```python
from build123d import *

# Parameters (mm, degrees)
F0_W     = 45.7
F0_H     = 4
F1_DEPTH = 1
F0_W_2   = 13.3
F0_H_2   = 2
F0_H_3   = 8.5
F0_W_3   = 2
F2_DEPTH = 2.5
F3_DEPTH = 5
F4_DEPTH = 8


with BuildPart() as f1:
    # F0 (on Top) → F1 (new body)
    with BuildSketch(Plane.XY):
        Polygon((59, 16.5), (59, 24.5), (45.7, 24.5), (45.7, 20.5), (45.7, 16.5), align=None)
        with Locations((22.85, 22.5)):
            Rectangle(F0_W, F0_H)
    extrude(amount=F1_DEPTH)



with BuildPart() as f1b:
    # F0 (on Top) → F1, piece 2 (new body)
    with BuildSketch(Plane.XY):
        Polygon((59, 0), (59, 8), (45.7, 8), (45.7, 4), (45.7, 0), align=None)
        with Locations((22.85, 2)):
            Rectangle(F0_W, F0_H)
    extrude(amount=F1_DEPTH)


with BuildPart() as f1_1:
    add(f1.part)

    add(f1b.part)  # F2 merges F1b
    # F0 (on Top) → F2 (join)
    with BuildSketch(Plane.XY):
        with Locations((52.35, 25.5)):
            Rectangle(F0_W_2, F0_H_2)
        with Locations((52.35, 12.25)):
            Rectangle(F0_W_2, F0_H_3)
        with Locations((52.35, -1)):
            Rectangle(F0_W_2, F0_H_2)
        with Locations((60, 12.25)):
            Rectangle(F0_W_3, F0_H_3)
        Polygon((61, -2), (61, 8), (59, 8), (59, 0), (59, -2), align=None)
        Polygon((61, 26.5), (59, 26.5), (59, 24.5), (59, 16.5), (61, 16.5), align=None)
    extrude(amount=F2_DEPTH)

    # F0 (on Top) → F3 (join)
    with BuildSketch(Plane.XY):
        Polygon((45.7, 8), (45.7, 16.5), (45.7, 20.5), (0, 20.5), (0, 4), (45.7, 4), align=None)
    extrude(amount=F3_DEPTH)

    # F0 (on Top) → F4 (join)
    with BuildSketch(Plane.XY):
        Polygon((45.7, 24.5), (45.7, 26.5), (-2, 26.5), (-2, -2), (45.7, -2), (45.7, 0), (0, 0), (0, 4), (0, 20.5), (0, 24.5), align=None)
    extrude(amount=F4_DEPTH)


solid = f1_1.part
```
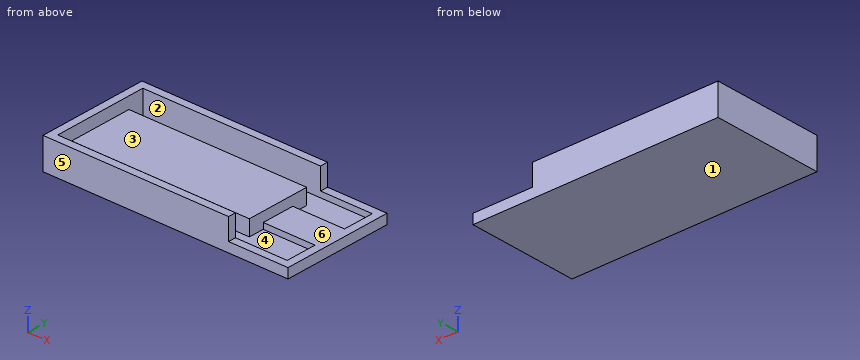
Check sheet for the modelled part. Datum: model origin and axes. Units: mm. Face numbers are marked on the shaded views. A direction names the side the tool comes from. Round coordinates to 2 decimals unless told otherwise and drop trailing zeros. Order: outer loops, then holes, each group sorted by start corner. A loop starts at its lowest first (then second) coordinate and runs counter-clockwise, first axis right, second up. Notation, with made-up numbers: M 27.25,55.5 L 43.25,55.5 A12 cw 43.25,63.5 Z; hole C -1,16.25 d6. An arc over 180 degrees is marked long. Answer in a Markdown table with one row per item.
(1) Section check A-A on z = 6.25. Record the boundary of the cut face in (x, y), plus the area to 3 significant figures.
Findings:
| item | result |
|---|---|
| outline | M -2,-2 L 45.7,-2 L 45.7,0 L 0,0 L 0,24.5 L 45.7,24.5 L 45.7,26.5 L -2,26.5 Z |
| area | 240 mm^2 |
(2) Section check D-D on x = 52.5. Record the boundary of the cut face in (y, z).
Findings:
| item | result |
|---|---|
| outline | M -2,0 L 26.5,0 L 26.5,2.5 L 24.5,2.5 L 24.5,1 L 16.5,1 L 16.5,2.5 L 8,2.5 L 8,1 L 0,1 L 0,2.5 L -2,2.5 Z |
(3) Draft check along Y on the marked faces 4, 5 and 6. Enter one of: +Y half, -Y half, draft (parallel to the pull), parting line (faces both ways), or undercut.
Findings:
| item | result |
|---|---|
| face 4 | undercut |
| face 5 | -Y half |
| face 6 | draft |
(4) Section check C-C on x = 21. Record the boundary of the cut face in (y, z).
Findings:
| item | result |
|---|---|
| outline | M -2,0 L 26.5,0 L 26.5,8 L 24.5,8 L 24.5,1 L 20.5,1 L 20.5,5 L 4,5 L 4,1 L 0,1 L 0,8 L -2,8 Z |
(5) Set-up check for the marked faces 1, 2 and 3: record each of +Z, -Z, +X, -X, +Y, -Y from which the full face is reachable in a straight line by a thin tool's end or side.
Findings:
| item | result |
|---|---|
| face 1 | -Z, +X, -X, +Y, -Y |
| face 2 | +Z |
| face 3 | +Z, +X |
(6) Section check B-B on y = 13. Record the boundary of the cut face in (x, z).
Findings:
| item | result |
|---|---|
| outline | M -2,0 L 61,0 L 61,2.5 L 45.7,2.5 L 45.7,5 L 0,5 L 0,8 L -2,8 Z |
(7) Material ranges on line 1 along Y through (x, z) = (28, 2); line 2 along Y through (x, z) = (1.5, 6); line 3 along Z through (x, y) = (54.5, 25), recorded low to high. Write a range as from..to.
Findings:
| item | result |
|---|---|
| line 1 | y = -2..0, 4..20.5, 24.5..26.5 |
| line 2 | y = -2..0, 24.5..26.5 |
| line 3 | z = 0..2.5 |
(8) Gauge pin test, flat ends, axial feed: pin 1 (1.6 mm diameter, centred on y = -0.5, z = 6, fed in from +X); pin 2 (6.5 mm diameter, centred on x = 19, y = 19, fed in from +Z); pin 3 (4 mm diameter, centred on x = 48, z = 5.5, fed in from -Y); pin 4 (7.5 mm diameter, centred on x = 56.5, y = 6, fed in from +Z). Record the tip position at first contact, or that the pin passes through.
Findings:
| item | result |
|---|---|
| pin 1 | stops at x = 45.7 |
| pin 2 | stops at z = 5 |
| pin 3 | passes through |
| pin 4 | stops at z = 2.5 |
